Geometry: final body of the model. Coordinates: model frame, mm. Face numbers are marked on the shaded views. A direction names the side the tool comes from. Round coordinates to 2 decimals unless told otherwise and drop trailing zeros. Write each loop counter-clockwise with the first axis right and the second up, starting at its lowest first coordinate (ties: lowest second). Pieces come first, ordered by that corner, then holes. Notation, with made-up numbers: M 41,46.25 L 88,46.25 A9 ccw 88,51.25 Z; hole C -11,43 d1. An arc over 180 degrees is marked long. Use one line per item in the form item = value. Start each with the question number.
Item 1: Ray query, probe 1 along Z at (x, y) = (11, 4); probe 2 along Z at (x, y) = (6.5, 35); probe 3 along Z at (x, y) = (19.5, -2.5). Return the intervals inside material, ascending.
Item 2: Section query D-D (y = 23.5). Return loops of the section in (x, z).
Item 3: Section query C-C (y = 38.5). Return loops of the section in (x, z).
Item 4: Section query B-B (y = 8). Return loops of the section in (x, z).
Item 5: Section query A-A (x = 22.5). Return loops of the section in (y, z).
Item 6: Pull-direction query (Y, two-part tool) for the marked faces 3, 4 and 5; classes: pulls with the +Y half, pulls with the -Y half, needs draft (parallel to the pull), parting line crosses it, or undercut.
Item 7: Pin query (flat end, axial travel): pin 1 Ø10 at (x, z) = (28, 12.5) entering from -Y; pin 2 Ø12 at (x, y) = (10, 29) entering from -Z; pin 3 Ø1 at (x, y) = (26.5, 10) entering from -Z. Return the tip coordinate at first contact, or that it passes through.
Item 8: Reachability of the marked faces 1 and 2 from +Z, -Z, +X, -X, +Y, -Y: full face, straight path, thin tool, end or side. Return the list, or none.
from build123d import *

# Parameters (mm, degrees)
F1_DEPTH = 50.8
F2_R     = 2.7639393044
F2_R_2   = 8.6653307134
F3_DEPTH = 79.502
F4_T     = -2.54


with BuildPart() as f1:
    # F0 (on Right) → F1 (new body)
    with BuildSketch(Plane.YZ):
        with BuildLine():
            ThreePointArc((0, -8.1618588303), (5.771305726, -5.771305726), (8.1618588303, 0))
            ThreePointArc((8.1618588303, 0), (5.771305726, 5.771305726), (0, 8.1618588303))
            ThreePointArc((0, 8.1618588303), (-8.1618588303, 0), (0, -8.1618588303))
        make_face()
        with BuildLine():
            ThreePointArc((57.4225941824, 0), (50.5917612932, 13.9660503324), (35.3738057369, 17.1479787622))
            ThreePointArc((35.3738057369, 17.1479787622), (22.0373280273, 0), (35.3738057369, -17.1479787622))
            ThreePointArc((35.3738057369, -17.1479787622), (50.5917612932, -13.9660503324), (57.4225941824, 0))
        make_face()
        with BuildLine():
            ThreePointArc((0, 8.1618588303), (5.771305726, 5.771305726), (8.1618588303, 0))
            ThreePointArc((8.1618588303, 0), (5.771305726, -5.771305726), (0, -8.1618588303))
            Line((0, -8.1618588303), (35.3738057369, -17.1479787622))
            ThreePointArc((35.3738057369, -17.1479787622), (22.0373280273, 0), (35.3738057369, 17.1479787622))
            Line((35.3738057369, 17.1479787622), (0, 8.1618588303))
        make_face()
    extrude(amount=F1_DEPTH)

    # F2 (on face) → F3 (cut)
    with BuildSketch(Plane(origin=(0, 0, 0), x_dir=(0, -1, 0), z_dir=(-1, 0, 0))):
        Circle(F2_R)
        with Locations((-39.7299611049, 0)):
            Circle(F2_R_2)
    extrude(amount=-F3_DEPTH, mode=Mode.SUBTRACT)

    # F4
    f4_openings = [f1.faces().sort_by_distance(p)[0] for p in [
        (0, 26.679648, 0),
    ]]
    offset(amount=F4_T, openings=f4_openings, kind=Kind.INTERSECTION)


solid = f1.part
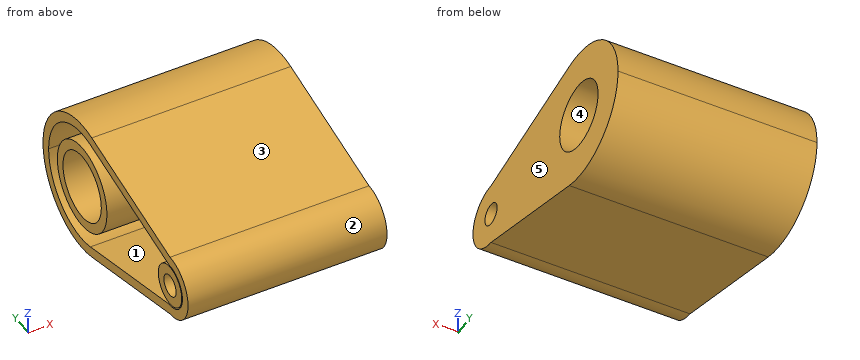
Working result:
q1.probe_1 = -9.18 to -6.56, -3.48 to 3.48, 6.56 to 9.18
q1.probe_2 = -17.05 to -14.43, -10.16 to -7.26, 7.26 to 10.16, 14.43 to 17.05
q1.probe_3 = -7.77 to -5.04, -4.68 to -1.18, 1.18 to 4.68, 5.04 to 7.77
q2.outline = M 0,-14.13 L 50.8,-14.13 L 50.8,14.13 L 0,14.13 L 0,11.51 L 48.26,11.51 L 48.26,-11.51 L 0,-11.51 Z
q3.outline = M 0,-17.65 L 50.8,-17.65 L 50.8,-8.58 L 0,-8.58 L 0,-11.14 L 48.26,-11.14 L 48.26,-15.1 L 0,-15.1 Z; M 0,8.58 L 50.8,8.58 L 50.8,17.65 L 0,17.65 L 0,15.1 L 48.26,15.1 L 48.26,11.14 L 0,11.14 Z
q4.outline = M 0,-10.19 L 50.8,-10.19 L 50.8,10.19 L 0,10.19 L 0,7.57 L 48.26,7.57 L 48.26,-7.57 L 0,-7.57 Z
q5.outline = C 0,0 d10.61; M 0,-8.16 L 35.37,-17.15 A17.69 ccw long 35.37,17.15 L 0,8.16 A8.16 ccw Z; C 39.73,0 d22.41; hole C 0,0 d5.53; hole M 0.29,-5.61 L 36,-14.69 A15.15 ccw long 36,14.69 L 0.29,5.61 A5.62 ccw long Z; hole C 39.73,0 d17.33
q6.face_3 = pulls with the -Y half
q6.face_4 = undercut
q6.face_5 = needs draft
q7.pin_1 = -3.22
q7.pin_2 = -17.05
q7.pin_3 = -10.83
q8.face_1 = -X
q8.face_2 = +X, -X, -Y
